from build123d import *
from build123d.topology import SkipClean

# Parameters (mm, degrees)
SKETCH_1_R               = 45
SKETCH_1_R_2             = 37
EXTRUDE_1_DEPTH          = 8
EXTRUDE_START            = 4
SKETCH_2_R               = 47.5
SKETCH_2_R_2             = 37
EXTRUDE_2_DEPTH          = 4
EXTRUDE_START_2          = -8
SKETCH_2_2_R             = 47.5
SKETCH_2_2_R_2           = 37
EXTRUDE_5_DEPTH          = 3
CUT_EXTRUDE_1_DEPTH      = 69.82949949
CUT_EXTRUDE_1_DEPTH_BACK = 69.82949949
SKETCH_3_R               = 2.1
EXTRUDE_START_3          = 8
SKETCH_4_R               = 37
SKETCH_4_R_2             = 8
SKETCH_4_R_3             = 1.6
SKETCH_4_R_4             = 1.3
EXTRUDE_3_DEPTH          = 3
CUT_EXTRUDE_START        = 12
CUT_EXTRUDE_3_DEPTH      = 3
CUT_EXTRUDE_4_DEPTH      = 69.82949949
PATTERN_START            = 8
PATTERN_CIRCULAR_1_DEPTH = 3


# Read off the part's stored shape, not the designer's step: 切除-拉伸3, 阵列(圆周)1
with BuildPart() as part:
    # 草图1 → 凸台-拉伸1 (new body)
    with BuildSketch(Plane.XY):
        Circle(SKETCH_1_R)
        Circle(SKETCH_1_R_2, mode=Mode.SUBTRACT)
    extrude(amount=EXTRUDE_1_DEPTH)

    # 草图2 → 凸台-拉伸2 (add)
    with SkipClean():  # the faces are left unmerged after this step: merging them gives an invalid solid
        with BuildSketch(Plane(origin=(0, 0, 0), x_dir=(-1, 0, 0), z_dir=(0, 0, -1)).offset(EXTRUDE_START)):
            Circle(SKETCH_2_R)
            Circle(SKETCH_2_R_2, mode=Mode.SUBTRACT)
        extrude(amount=-EXTRUDE_2_DEPTH)

    # 草图2<2> → 凸台-拉伸5 (add)
    with BuildSketch(Plane(origin=(0, 0, 0), x_dir=(-1, 0, 0), z_dir=(0, 0, -1)).offset(EXTRUDE_START_2)):
        Circle(SKETCH_2_2_R)
        Circle(SKETCH_2_2_R_2, mode=Mode.SUBTRACT)
    extrude(amount=-EXTRUDE_5_DEPTH)

    # 草图3 → 切除-拉伸1 (cut, two sides: drawn at the far end of the back side and taken through both)
    with BuildSketch(Plane.XY.offset(11).offset(-CUT_EXTRUDE_1_DEPTH_BACK)):
        with Locations((0, 41)):
            Circle(SKETCH_3_R)
        with Locations((15.690020727, 37.879060833)):
            Circle(SKETCH_3_R)
        with Locations((28.991378029, 28.991378029)):
            Circle(SKETCH_3_R)
        with Locations((37.879060833, 15.690020727)):
            Circle(SKETCH_3_R)
        with Locations((41, 0)):
            Circle(SKETCH_3_R)
        with Locations((37.879060833, -15.690020727)):
            Circle(SKETCH_3_R)
        with Locations((28.991378029, -28.991378029)):
            Circle(SKETCH_3_R)
        with Locations((15.690020727, -37.879060833)):
            Circle(SKETCH_3_R)
        with Locations((0, -41)):
            Circle(SKETCH_3_R)
        with Locations((-15.690020727, -37.879060833)):
            Circle(SKETCH_3_R)
        with Locations((-28.991378029, -28.991378029)):
            Circle(SKETCH_3_R)
        with Locations((-37.879060833, -15.690020727)):
            Circle(SKETCH_3_R)
        with Locations((-41, 0)):
            Circle(SKETCH_3_R)
        with Locations((-37.879060833, 15.690020727)):
            Circle(SKETCH_3_R)
        with Locations((-28.991378029, 28.991378029)):
            Circle(SKETCH_3_R)
        with Locations((-15.690020727, 37.879060833)):
            Circle(SKETCH_3_R)
    extrude(amount=CUT_EXTRUDE_1_DEPTH + CUT_EXTRUDE_1_DEPTH_BACK, mode=Mode.SUBTRACT)

    # 草图4 → 凸台-拉伸3 (add)
    with BuildSketch(Plane.XY.offset(EXTRUDE_START_3)):
        with Locations(Location((0, 0, 0), (0, 0, 180))):
            Circle(SKETCH_4_R)
        Circle(SKETCH_4_R_2, mode=Mode.SUBTRACT)
        with Locations((20, 0)):
            Circle(SKETCH_4_R_3, mode=Mode.SUBTRACT)
        with Locations((10, -17.320508076)):
            Circle(SKETCH_4_R_3, mode=Mode.SUBTRACT)
        with Locations((-10, -17.320508076)):
            Circle(SKETCH_4_R_3, mode=Mode.SUBTRACT)
        with Locations((12.5, 0)):
            Circle(SKETCH_4_R_4, mode=Mode.SUBTRACT)
        with Locations((-20, 0)):
            Circle(SKETCH_4_R_3, mode=Mode.SUBTRACT)
        with Locations((-10, 17.320508076)):
            Circle(SKETCH_4_R_3, mode=Mode.SUBTRACT)
        with Locations((10, 17.320508076)):
            Circle(SKETCH_4_R_3, mode=Mode.SUBTRACT)
        with Locations((6.25, -10.825317547)):
            Circle(SKETCH_4_R_4, mode=Mode.SUBTRACT)
        with Locations((-6.25, -10.825317547)):
            Circle(SKETCH_4_R_4, mode=Mode.SUBTRACT)
        with Locations((-12.5, 0)):
            Circle(SKETCH_4_R_4, mode=Mode.SUBTRACT)
        with Locations((-6.25, 10.825317547)):
            Circle(SKETCH_4_R_4, mode=Mode.SUBTRACT)
        with Locations((6.25, 10.825317547)):
            Circle(SKETCH_4_R_4, mode=Mode.SUBTRACT)
    extrude(amount=EXTRUDE_3_DEPTH)

    # 切除-拉伸3 outline → 切除-拉伸3 (cut)
    with BuildSketch(Plane.XY.offset(-4).offset(CUT_EXTRUDE_START)):
        with BuildLine():
            Line((-4.514852619, 25.605001578), (-6.424982574, 36.437886861))
            ThreePointArc((-6.424982574, 36.437886861), (-18.5, 32.04293994), (-28.343644395, 23.783141558))
            Line((-28.343644395, 23.783141558), (-19.917155521, 16.712477852))
            ThreePointArc((-19.917155521, 16.712477852), (-13, 22.516660498), (-4.514852619, 25.605001578))
        make_face()
        with BuildLine():
            ThreePointArc((6.424982574, -36.437886861), (18.5, -32.04293994), (28.343644395, -23.783141558))
            Line((28.343644395, -23.783141558), (19.917155521, -16.712477852))
            ThreePointArc((19.917155521, -16.712477852), (13, -22.516660498), (4.514852619, -25.605001578))
            Line((4.514852619, -25.605001578), (6.424982574, -36.437886861))
        make_face()
    extrude(amount=CUT_EXTRUDE_3_DEPTH, mode=Mode.SUBTRACT)

    # 草图8 → Cut-Extrude 4 (cut, through all)
    with BuildSketch(Plane.XY.offset(11)):
        with BuildLine():
            ThreePointArc((4.514852619, -25.605001578), (-19.917155521, -16.712477852), (-24.43200814, 8.892523726))
            Line((-24.43200814, 8.892523726), (-26.311393382, 9.576564013))
            ThreePointArc((-26.311393382, 9.576564013), (-21.449244407, -17.998053071), (4.862148975, -27.574617084))
            Line((4.862148975, -27.574617084), (4.514852619, -25.605001578))
        make_face()
        with BuildLine():
            ThreePointArc((-28.343644395, 23.783141558), (-34.768626969, -12.654745303), (-6.424982574, -36.437886861))
            Line((-6.424982574, -36.437886861), (-6.077686218, -34.468271355))
            ThreePointArc((-6.077686218, -34.468271355), (-32.889241728, -11.970705016), (-26.811555509, 22.497566339))
            Line((-26.811555509, 22.497566339), (-28.343644395, 23.783141558))
        make_face()
    extrude(amount=-CUT_EXTRUDE_4_DEPTH, mode=Mode.SUBTRACT)


with BuildPart() as cut_extrude_4_kept_piece:
    # of the separate pieces the step leaves, the one the design keeps (cut_extrude_4_pieces_kept)
    add(part.part.solids().sort_by_distance((45, 0, 8))[0])

    # 阵列(圆周)1 outline → 阵列(圆周)1 (cut)
    with BuildSketch(Plane.XY.offset(PATTERN_START)):
        with BuildLine():
            ThreePointArc((28.343644395, -23.783141558), (34.768626969, 12.654745303), (6.424982574, 36.437886861))
            Line((6.424982574, 36.437886861), (6.077686218, 34.468271355))
            ThreePointArc((6.077686218, 34.468271355), (32.889241728, 11.970705017), (26.811555509, -22.497566339))
            Line((26.811555509, -22.497566339), (28.343644395, -23.783141558))
        make_face()
        with BuildLine():
            ThreePointArc((26.311393382, -9.576564013), (21.449244407, 17.998053071), (-4.862148975, 27.574617084))
            Line((-4.862148975, 27.574617084), (-4.514852619, 25.605001578))
            ThreePointArc((-4.514852619, 25.605001578), (19.917155521, 16.712477852), (24.43200814, -8.892523726))
            Line((24.43200814, -8.892523726), (26.311393382, -9.576564013))
        make_face()
    extrude(amount=PATTERN_CIRCULAR_1_DEPTH, mode=Mode.SUBTRACT)


solid = cut_extrude_4_kept_piece.part
Here's how the part is built. I have some questions about the finished solid (model axes, mm). Coordinates: 2 decimals unless noted, no trailing zeros.
Item 1: If we mould it in two halves opening along X, with no side actions, what happens to faces 1 (the flat face through (-42, -17, 0)), 2 (the cylindrical face through (28.72, -26.91, 3.39)), 3 (the cylindrical face through (8.4, -17.3, 9.5))? For each: +X half, -X half, draft (parallel to the pull), parting line (faces both ways), or undercut.
Item 2: I want a section at A-A on z = 6.5. Count the separate pieces of the cut face and the enclosed holes in it, and give its area (3 significant figures).
Item 3: If I drill on line 1 (Y direction, x = -14, z = -0.5); line 2 (X direction, y = 28, z = -1.5); line 3 (Y direction, x = 30, z = 8.5), over which ranges is the centre line in solid material (lowest first)?
Item 4: Will these pins go through, and if not, where does the flat tip stop? pin 1 (3 mm diameter, centred on x = -10, y = -17.32, fed in from -Z); pin 2 (6.5 mm diameter, centred on x = -41, y = 0, fed in from +Z); pin 3 (6 mm diameter, centred on x = -7, z = -0.5, fed in from +Y); pin 4 (8 mm diameter, centred on y = 7, z = 3, fed in from -X).
Findings below:
1. face 1: draft
1. face 2: undercut
1. face 3: undercut
2. separate pieces: 1
2. enclosed holes: 17
2. area: 1,840 mm2
3. line 1: y = -45.39 to -39.13, -36.63 to -34.25, 34.25 to 36.63, 39.13 to 45.39
3. line 2: x = -38.37 to -30.84, -27.14 to -24.19, 24.19 to 27.14, 30.84 to 38.37
3. line 3: y = -36.83 to -30.83, -27.15 to -21.66, -18.03 to 18.03, 21.66 to 27.15, 30.83 to 36.83
4. pin 1: passes through
4. pin 2: stops at z = 11
4. pin 3: stops at y = 47.33
4. pin 4: stops at x = -47.3
